```python
from build123d import *

# Parameters (mm, degrees)
SKETCH1_W           = 54
SKETCH1_H           = 29
BOSS_EXTRUDE1_DEPTH = 50
SHELL1_T            = -1.25
SKETCH2_W           = 35.25
SKETCH2_H           = 21
CUT_EXTRUDE1_DEPTH  = 51
CUT_EXTRUDE2_REACH  = 56
SKETCH3_W           = 12
SKETCH3_H           = 7.5
CUT_EXTRUDE3_REACH  = 52
SKETCH4_W           = 13
SKETCH4_H           = 1.5
CUT_EXTRUDE4_REACH  = 31
SKETCH6_W           = 15.64520267
SKETCH6_H           = 1.830091839
SKETCH6_W_2         = 22.646740458
SKETCH6_H_2         = 2.116515958
SKETCH6_W_3         = 26.646589607
SKETCH6_H_3         = 1.98929613
SKETCH6_H_4         = 1.878154188
SKETCH6_H_5         = 1.86823604
SKETCH6_H_6         = 1.784322078
SKETCH6_H_7         = 1.716719878


with BuildPart() as part:
    # Sketch1 → Boss-Extrude1 (new body)
    with BuildSketch(Plane(origin=(0, 0, 0), x_dir=(1, 0, 0), z_dir=(0, 1, 0))):
        Rectangle(SKETCH1_W, SKETCH1_H)
    extrude(amount=BOSS_EXTRUDE1_DEPTH)

    # Shell1
    shell1_openings = [part.faces().sort_by_distance(p)[0] for p in [
        (0, 50, 0),
    ]]
    offset(amount=SHELL1_T, openings=shell1_openings, kind=Kind.INTERSECTION)

    # Sketch2 → Cut-Extrude1 (cut, through all)
    with BuildSketch(Plane.XZ):
        with Locations((-6.625, 0)):
            Rectangle(SKETCH2_W, SKETCH2_H)
    extrude(amount=-CUT_EXTRUDE1_DEPTH, mode=Mode.SUBTRACT)

    # Sketch3 → Cut-Extrude2 (cut, up to next)
    with BuildSketch(Plane(origin=(27, 0, 0), x_dir=(0, 0, -1), z_dir=(1, 0, 0)), mode=Mode.PRIVATE) as cut_extrude2_sk1:
        with Locations((0, 6.75)):
            Rectangle(SKETCH3_W, SKETCH3_H)
    cut_extrude2_tool1 = extrude(cut_extrude2_sk1.sketch, amount=-CUT_EXTRUDE2_REACH, mode=Mode.PRIVATE) & part.part
    add(cut_extrude2_tool1.solids().sort_by_distance((27, 6.75, 0))[0], mode=Mode.SUBTRACT)

    # Sketch4 → Cut-Extrude3 (cut, up to next)
    with BuildSketch(Plane.XZ, mode=Mode.PRIVATE) as cut_extrude3_sk1:
        with Locations((-6.625, 11.25)):
            Rectangle(SKETCH4_W, SKETCH4_H)
    cut_extrude3_tool1 = extrude(cut_extrude3_sk1.sketch, amount=-CUT_EXTRUDE3_REACH, mode=Mode.PRIVATE) & part.part
    add(cut_extrude3_tool1.solids().sort_by_distance((-6.625, 0, 11.25))[0], mode=Mode.SUBTRACT)

    # Sketch6 → Cut-Extrude4 (cut, up to next)
    with BuildSketch(Plane(origin=(0, 0, -14.5), x_dir=(-1, 0, 0), z_dir=(0, 0, -1)), mode=Mode.PRIVATE) as cut_extrude4_sk1:
        with Locations((-9.330453993, 19.365591302)):
            Rectangle(SKETCH6_W, SKETCH6_H)
    cut_extrude4_tool1 = extrude(cut_extrude4_sk1.sketch, amount=-CUT_EXTRUDE4_REACH, mode=Mode.PRIVATE) & part.part
    add(cut_extrude4_tool1.solids().sort_by_distance((9.330454, 19.365591, -14.5))[0], mode=Mode.SUBTRACT)
    # Sketch6 → Cut-Extrude4 (cut, up to next)
    with BuildSketch(Plane(origin=(0, 0, -14.5), x_dir=(-1, 0, 0), z_dir=(0, 0, -1)), mode=Mode.PRIVATE) as cut_extrude4_sk2:
        with Locations((-9.158424139, 23.200549922)):
            Rectangle(SKETCH6_W_2, SKETCH6_H_2)
    cut_extrude4_tool2 = extrude(cut_extrude4_sk2.sketch, amount=-CUT_EXTRUDE4_REACH, mode=Mode.PRIVATE) & part.part
    add(cut_extrude4_tool2.solids().sort_by_distance((9.158424, 23.20055, -14.5))[0], mode=Mode.SUBTRACT)
    # Sketch6 → Cut-Extrude4 (cut, up to next)
    with BuildSketch(Plane(origin=(0, 0, -14.5), x_dir=(-1, 0, 0), z_dir=(0, 0, -1)), mode=Mode.PRIVATE) as cut_extrude4_sk3:
        with Locations((-8.981382512, 27.470306386)):
            Rectangle(SKETCH6_W_3, SKETCH6_H_3)
    cut_extrude4_tool3 = extrude(cut_extrude4_sk3.sketch, amount=-CUT_EXTRUDE4_REACH, mode=Mode.PRIVATE) & part.part
    add(cut_extrude4_tool3.solids().sort_by_distance((8.981383, 27.470306, -14.5))[0], mode=Mode.SUBTRACT)
    # Sketch6 → Cut-Extrude4 (cut, up to next)
    with BuildSketch(Plane(origin=(0, 0, -14.5), x_dir=(-1, 0, 0), z_dir=(0, 0, -1)), mode=Mode.PRIVATE) as cut_extrude4_sk4:
        with Locations((-8.981382512, 30.885196162)):
            Rectangle(SKETCH6_W_3, SKETCH6_H_4)
    cut_extrude4_tool4 = extrude(cut_extrude4_sk4.sketch, amount=-CUT_EXTRUDE4_REACH, mode=Mode.PRIVATE) & part.part
    add(cut_extrude4_tool4.solids().sort_by_distance((8.981383, 30.885196, -14.5))[0], mode=Mode.SUBTRACT)
    # Sketch6 → Cut-Extrude4 (cut, up to next)
    with BuildSketch(Plane(origin=(0, 0, -14.5), x_dir=(-1, 0, 0), z_dir=(0, 0, -1)), mode=Mode.PRIVATE) as cut_extrude4_sk5:
        with Locations((-9.158424139, 34.324467927)):
            Rectangle(SKETCH6_W_2, SKETCH6_H_5)
    cut_extrude4_tool5 = extrude(cut_extrude4_sk5.sketch, amount=-CUT_EXTRUDE4_REACH, mode=Mode.PRIVATE) & part.part
    add(cut_extrude4_tool5.solids().sort_by_distance((9.158424, 34.324468, -14.5))[0], mode=Mode.SUBTRACT)
    # Sketch6 → Cut-Extrude4 (cut, up to next)
    with BuildSketch(Plane(origin=(0, 0, -14.5), x_dir=(-1, 0, 0), z_dir=(0, 0, -1)), mode=Mode.PRIVATE) as cut_extrude4_sk6:
        with Locations((-9.158424139, 37.995559626)):
            Rectangle(SKETCH6_W_2, SKETCH6_H_6)
    cut_extrude4_tool6 = extrude(cut_extrude4_sk6.sketch, amount=-CUT_EXTRUDE4_REACH, mode=Mode.PRIVATE) & part.part
    add(cut_extrude4_tool6.solids().sort_by_distance((9.158424, 37.99556, -14.5))[0], mode=Mode.SUBTRACT)
    # Sketch6 → Cut-Extrude4 (cut, up to next)
    with BuildSketch(Plane(origin=(0, 0, -14.5), x_dir=(-1, 0, 0), z_dir=(0, 0, -1)), mode=Mode.PRIVATE) as cut_extrude4_sk7:
        with Locations((-9.330453993, 41.439907402)):
            Rectangle(SKETCH6_W, SKETCH6_H_7)
    cut_extrude4_tool7 = extrude(cut_extrude4_sk7.sketch, amount=-CUT_EXTRUDE4_REACH, mode=Mode.PRIVATE) & part.part
    add(cut_extrude4_tool7.solids().sort_by_distance((9.330454, 41.439907, -14.5))[0], mode=Mode.SUBTRACT)


solid = part.part
```
The model under review builds one solid part; all positions refer to its coordinate system, in mm. A direction names the side the tool comes from. Round coordinates to 2 decimals unless told otherwise and drop trailing zeros. Order: outer loops, then holes, each group sorted by start corner. A loop starts at its lowest first (then second) coordinate and runs counter-clockwise, first axis right, second up. Notation, with made-up numbers: (-31, 87.5) -> (22, 87.5) arc R23 cw to (22, 102.5) -> close; hole circle Ø8 at (24, 58). An arc over 180 degrees is marked (long way). One line per item, written item: value. Start each with the question number.
Q1. Take a section at D-D (y = 13). Write out the cut boundary in (x, z), and give its area (3 significant figures).
Q2. Take a section at C-C (z = -8.5). Write out the cut boundary in (x, y).
Q3. Take a section at A-A (z = -3.25). Write out the cut boundary in (x, y), and give its area (3 significant figures).
Q4. Take a section at B-B (x = -19). Write out the cut boundary in (y, z), and give its area (3 significant figures).
Q5. Mouldability with a two-part tool opening along X and no side actions: class faces 1 (the face through (-27, 25, 0)), 2 (the face through (9, 42.298, -14)), 3 (the face through (26, 7, 6)), 4 (the face through (9, 38.888, -14)) as released by +X, released by -X, zero draft, split by the parting line, or undercut.
Q6. Wall thickness on line 1 (Z direction, x = -6, y = 43); line 2 (X direction, y = 18, z = 6.25); line 3 (Y direction, x = 18.5, z = -4): over which ranges is each line inside the solid? List them lowest first.
Q7. Machinability: for faces 5 (the face through (0, 25, -13.25)), 6 (the face through (-7, 1, 12)), 7 (the face through (1.508, 41, -14)), 8 (the face through (26, 7, -6)), which of the approach directions +Z, -Z, +X, -X, +Y, -Y give a long, thin tool a straight path to every point of the face, cutting with its end or side? Answer none if there is none.
Reported:
1. outline: (-27, -14.5) -> (27, -14.5) -> (27, 14.5) -> (-27, 14.5) -> close; hole (-25.75, -13.25) -> (25.75, -13.25) -> (25.75, 13.25) -> (-25.75, 13.25) -> close
1. area: 201 mm2
2. outline: (-27, 0) -> (-24.25, 0) -> (-24.25, 1.25) -> (-25.75, 1.25) -> (-25.75, 50) -> (-27, 50) -> close; (11, 0) -> (27, 0) -> (27, 50) -> (25.75, 50) -> (25.75, 1.25) -> (11, 1.25) -> close
3. outline: (-27, 0) -> (-24.25, 0) -> (-24.25, 1.25) -> (-25.75, 1.25) -> (-25.75, 50) -> (-27, 50) -> close; (11, 0) -> (27, 0) -> (27, 3) -> (25.75, 3) -> (25.75, 1.25) -> (11, 1.25) -> close; (25.75, 10.5) -> (27, 10.5) -> (27, 50) -> (25.75, 50) -> close
3. area: 136 mm2
4. outline: (0, -14.5) -> (50, -14.5) -> (50, -13.25) -> (1.25, -13.25) -> (1.25, -10.5) -> (0, -10.5) -> close; (0, 10.5) -> (1.25, 10.5) -> (1.25, 13.25) -> (50, 13.25) -> (50, 14.5) -> (0, 14.5) -> close
4. area: 132 mm2
5. face 1: released by -X
5. face 2: undercut
5. face 3: zero draft
5. face 4: undercut
6. line 1: z = -14.5 to -13.25, 13.25 to 14.5
6. line 2: x = -27 to -25.75, 25.75 to 27
6. line 3: y = 0 to 1.25
7. face 5: +Y
7. face 6: +Y, -Y
7. face 7: -Z
7. face 8: +X
